```python
from build123d import *

# Parameters (mm, degrees)
Y_KSEKLIK_EKSTR_ZYON1_DEPTH             = 6
M3X0_5_HELISARMAL_IN_DI_LI_DELIK1_D     = 3.15
M3X0_5_HELISARMAL_IN_DI_LI_DELIK1_DEPTH = 7.5
M3X0_5_HELISARMAL_IN_DI_LI_DELIK1_TIP   = 0.946355475
M3X0_5_HELISARMAL_IN_DI_LI_DELIK2_D     = 3.15
M3X0_5_HELISARMAL_IN_DI_LI_DELIK2_DEPTH = 7.5
M3X0_5_HELISARMAL_IN_DI_LI_DELIK2_TIP   = 0.946355475
IZIM2_R                                 = 69
IZIM2_R_2                               = 59
KES_EKSTR_ZYON_NCE1_DEPTH               = 150


with BuildPart() as part:
    # Çizim1 → Yükseklik-Ekstrüzyon1 (new body)
    with BuildSketch(Plane.XY):
        Polygon((0, 20), (-10, 20), (-10, 30), (0, 30), (0, 90), (-10, 90), (-10, 100), (0, 100), (0, 120), (98.2, 120), (98.2, 100), (108.2, 100), (108.2, 90), (98.2, 90), (98.2, 30), (108.2, 30), (108.2, 20), (98.2, 20), (98.2, 0), (0, 0), align=None)
    extrude(amount=Y_KSEKLIK_EKSTR_ZYON1_DEPTH)

    # M3x0.5 Helisarmal İçin Dişli Delik1
    with Locations(Plane.ZY.offset(10)):
        with Locations((3, 25), (3, 95)):
            Hole(M3X0_5_HELISARMAL_IN_DI_LI_DELIK1_D / 2, depth=M3X0_5_HELISARMAL_IN_DI_LI_DELIK1_DEPTH)
            with Locations((0, 0, -(M3X0_5_HELISARMAL_IN_DI_LI_DELIK1_DEPTH + M3X0_5_HELISARMAL_IN_DI_LI_DELIK1_TIP / 2))):  # 118° drill point
                Cone(0, M3X0_5_HELISARMAL_IN_DI_LI_DELIK1_D / 2, M3X0_5_HELISARMAL_IN_DI_LI_DELIK1_TIP, mode=Mode.SUBTRACT)

    # M3x0.5 Helisarmal İçin Dişli Delik2
    with Locations(Plane(origin=(108.2, 0, 0), x_dir=(0, 0, -1), z_dir=(1, 0, 0))):
        with Locations((-3, 25), (-3, 95)):
            Hole(M3X0_5_HELISARMAL_IN_DI_LI_DELIK2_D / 2, depth=M3X0_5_HELISARMAL_IN_DI_LI_DELIK2_DEPTH)
            with Locations((0, 0, -(M3X0_5_HELISARMAL_IN_DI_LI_DELIK2_DEPTH + M3X0_5_HELISARMAL_IN_DI_LI_DELIK2_TIP / 2))):  # 118° drill point
                Cone(0, M3X0_5_HELISARMAL_IN_DI_LI_DELIK2_D / 2, M3X0_5_HELISARMAL_IN_DI_LI_DELIK2_TIP, mode=Mode.SUBTRACT)

    # Çizim2 → Kes-Ekstrüzyon-İnce1 (cut)
    with BuildSketch(Plane(origin=(0, 120, 0), x_dir=(1, 0, 0), z_dir=(0, 1, 0))):
        with Locations((49.1, -3)):
            Circle(IZIM2_R)
        with Locations((49.1, -3)):
            Circle(IZIM2_R_2, mode=Mode.SUBTRACT)
    extrude(amount=-KES_EKSTR_ZYON_NCE1_DEPTH, mode=Mode.SUBTRACT)


solid = part.part
```
Here's how the part is built. I have some questions about the finished solid (model axes, mm). A direction names the side the tool comes from. Coordinates: 2 decimals unless noted, no trailing zeros. Order: outer loops, then holes, each group sorted by start corner. A loop starts at its lowest first (then second) coordinate and runs counter-clockwise, first axis right, second up.
Item 1: I'm going to push flat-ended pins straight in: pin 1 Ø1 at (y, z) = (83, 2) entering from -X; pin 2 Ø1.8 at (y, z) = (113, 1.5) entering from +X; pin 3 Ø3 at (x, z) = (101, 2) entering from -Y. Where does each tip first touch, or does it pass through?
Response values:
pin 1: stops at x = 0
pin 2: stops at x = 98.2
pin 3: stops at y = 20
Item 2: I need wall thicknesses on probe 1 along Y at (x, z) = (-5.75, 3) (3 decimals); probe 2 along Y at (x, z) = (101.5, 4); probe 3 along X at (y, z) = (10.5, 5.75). Which ranges of each line are inside material? Lowest first, please.
Response values:
probe 1: y = 20 to 23.425, 26.575 to 30, 90 to 93.425, 96.575 to 100
probe 2: y = 20 to 23.78, 26.22 to 30, 90 to 93.78, 96.22 to 100
probe 3: x = 0 to 98.2
Item 3: If we section it at A-A, the plane y = 84: List the corners of the cut face in (x, z) for me, then the cut area to 3 significant figures.
Response values:
outline: (0, 0) - (98.2, 0) - (98.2, 6) - (0, 6) - close
area: 589 mm2
Item 4: Which directions (+Z, -Z, +X, -X, +Y, -Y) give clear straight access to the entire face, cutting with the end or side of a thin tool? Please do faces 5 (the face through (103, 100, 3)), 6 (the face through (0, 110, 3)), 7 (the face through (98.2, 60, 3)), 8 (the face through (98.2, 10, 3)).
Response values:
face 5: +Z, -Z, +X, +Y
face 6: +Z, -Z, -X, +Y
face 7: +Z, -Z, +X
face 8: +Z, -Z, +X, -Y
Item 5: Thinking about a two-plate mould opening in Y: for faces 1 (the face through (104.348, 93.462, 2.659)), 2 (the face through (50, 0, 3)), 3 (the face through (-6.148, 93.462, 3.341)), 4 (the face through (0, 10, 3)), which applies, pulls with the +Y half, pulls with the -Y half, needs draft (parallel to the pull), parting line crosses it, or undercut?
Response values:
face 1: undercut
face 2: pulls with the -Y half
face 3: undercut
face 4: needs draft
